Could you check a few things on this model? Use its own coordinates, in mm. Give positions to 0.01 mm unless a question says otherwise; leave off trailing zeros. Write each loop counter-clockwise with the first axis right and the second up, starting at its lowest first coordinate (ties: lowest second). Pieces come first, ordered by that corner, then holes. Notation, with made-up numbers: (-30.5, 17) - (24.5, 17) arc R20 ccw to (24.5, 36) - close; hole circle Ø10 at (-20, 88). An arc over 180 degrees is marked (long way). Write item = value, one per line.
from build123d import *
from build123d import SkipClean  # not in build123d's __all__

# Parameters (mm, degrees)
F0_R      = 3.175
F1_DEPTH  = 127
F2_DEPTH  = 76.2
F3_DEPTH  = 71.12
F4_DEPTH  = 50.8
F5_DEPTH  = 45.72
F6_DEPTH  = 25.4
F7_DEPTH  = 20.32
F9_DEPTH  = 8.89
F10_DEPTH = 3.81
F12_DEPTH = 8.89
F13_DEPTH = 3.81
F15_DEPTH = 8.89
F16_DEPTH = 3.81
F17_DEPTH = 17.78


# Not quite as in the source:
# - after a boolean that leaves OpenCascade's solid faulty, fix() repairs it


with BuildPart() as f1:
    # F0 (on Top) → F1 (new body)
    with BuildSketch(Plane.XY):
        with BuildLine():
            ThreePointArc((7.6934750952, -1.6764), (7.8287386883, -0.8430459954), (7.874, 0))
            ThreePointArc((7.874, 0), (7.8574202107, 0.5107089515), (7.8077506647, 1.0192671673))
            ThreePointArc((7.8077506647, 1.0192671673), (5.6566372636, 5.4774383491), (1.27, 7.7709057387))
            ThreePointArc((1.27, 7.7709057387), (0, 7.874), (-1.27, 7.7709057387))
            ThreePointArc((-1.27, 7.7709057387), (-7.8735779463, 0.0815249862), (-1.430634249, -7.7429426994))
            ThreePointArc((-1.430634249, -7.7429426994), (-0.0815249862, -7.8735779463), (1.27, -7.7709057387))
            ThreePointArc((1.27, -7.7709057387), (5.4195683864, -5.7121059606), (7.6934750952, -1.6764))
        make_face()
        Circle(F0_R, mode=Mode.SUBTRACT)
    extrude(amount=F1_DEPTH)

    # F0 (on Top) → F2 (join)
    with BuildSketch(Plane.XY):
        with BuildLine():
            ThreePointArc((-1.27, 7.7709057387), (0, 7.874), (1.27, 7.7709057387))
            Line((1.27, 7.7709057387), (1.27, 12.3429057387))
            Line((1.27, 12.3429057387), (-1.27, 12.3429057387))
            Line((-1.27, 12.3429057387), (-1.27, 7.7709057387))
        make_face()
    extrude(amount=F2_DEPTH)

    # F0 (on Top) → F3 (cut)
    with BuildSketch(Plane.XY):
        with BuildLine():
            ThreePointArc((-1.27, 7.7709057387), (0, 7.874), (1.27, 7.7709057387))
            Line((1.27, 7.7709057387), (1.27, 12.3429057387))
            Line((1.27, 12.3429057387), (-1.27, 12.3429057387))
            Line((-1.27, 12.3429057387), (-1.27, 7.7709057387))
        make_face()
    with SkipClean():  # cleaning this boolean's faces spoils the solid; the shape is the same uncleaned
        extrude(amount=F3_DEPTH, mode=Mode.SUBTRACT)

    # F0 (on Top) → F4 (join)
    with BuildSketch(Plane.XY):
        with BuildLine():
            ThreePointArc((7.8077506647, 1.0192671673), (7.8574202107, 0.5107089515), (7.874, 0))
            ThreePointArc((7.874, 0), (7.8287386883, -0.8430459954), (7.6934750952, -1.6764))
            Line((7.6934750952, -1.6764), (12.2654750952, -1.6764))
            Line((12.2654750952, -1.6764), (12.2654750952, 0.8636))
            Line((12.2654750952, 0.8636), (7.8077506647, 1.0192671673))
        make_face()
    extrude(amount=F4_DEPTH)

    add(f1.part.fix(), mode=Mode.REPLACE)

    # F0 (on Top) → F5 (cut)
    with BuildSketch(Plane.XY):
        with BuildLine():
            ThreePointArc((7.8077506647, 1.0192671673), (7.8574202107, 0.5107089515), (7.874, 0))
            ThreePointArc((7.874, 0), (7.8287386883, -0.8430459954), (7.6934750952, -1.6764))
            Line((7.6934750952, -1.6764), (12.2654750952, -1.6764))
            Line((12.2654750952, -1.6764), (12.2654750952, 0.8636))
            Line((12.2654750952, 0.8636), (7.8077506647, 1.0192671673))
        make_face()
    with SkipClean():  # cleaning this boolean's faces spoils the solid; the shape is the same uncleaned
        extrude(amount=F5_DEPTH, mode=Mode.SUBTRACT)

    # F0 (on Top) → F6 (join)
    with BuildSketch(Plane.XY):
        with BuildLine():
            Line((1.27, -12.3429057387), (1.27, -7.7709057387))
            ThreePointArc((1.27, -7.7709057387), (-0.0815249862, -7.8735779463), (-1.430634249, -7.7429426994))
            Line((-1.430634249, -7.7429426994), (-1.27, -12.3429057387))
            Line((-1.27, -12.3429057387), (1.27, -12.3429057387))
        make_face()
    extrude(amount=F6_DEPTH)

    add(f1.part.fix(), mode=Mode.REPLACE)

    # F0 (on Top) → F7 (cut)
    with BuildSketch(Plane.XY):
        with BuildLine():
            Line((1.27, -12.3429057387), (1.27, -7.7709057387))
            ThreePointArc((1.27, -7.7709057387), (-0.0815249862, -7.8735779463), (-1.430634249, -7.7429426994))
            Line((-1.430634249, -7.7429426994), (-1.27, -12.3429057387))
            Line((-1.27, -12.3429057387), (1.27, -12.3429057387))
        make_face()
    with SkipClean():  # cleaning this boolean's faces spoils the solid; the shape is the same uncleaned
        extrude(amount=F7_DEPTH, mode=Mode.SUBTRACT)

    # F8 (on face) → F9 (join)
    with BuildSketch(Plane.XY.offset(76.2)):
        with BuildLine():
            Line((1.27, 12.3429057387), (-1.27, 12.3429057387))
            Line((-1.27, 12.3429057387), (-1.27, 7.7709057387))
            ThreePointArc((-1.27, 7.7709057387), (0, 7.874), (1.27, 7.7709057387))
            Line((1.27, 7.7709057387), (1.27, 12.3429057387))
        make_face()
    extrude(amount=F9_DEPTH)

    # F8 (on face) → F10 (cut)
    with BuildSketch(Plane.XY.offset(76.2)):
        with BuildLine():
            Line((1.27, 12.3429057387), (-1.27, 12.3429057387))
            Line((-1.27, 12.3429057387), (-1.27, 7.7709057387))
            ThreePointArc((-1.27, 7.7709057387), (0, 7.874), (1.27, 7.7709057387))
            Line((1.27, 7.7709057387), (1.27, 12.3429057387))
        make_face()
    with SkipClean():  # cleaning this boolean's faces spoils the solid; the shape is the same uncleaned
        extrude(amount=F10_DEPTH, mode=Mode.SUBTRACT)

    # F11 (on face) → F12 (join)
    with BuildSketch(Plane.XY.offset(50.8)):
        with BuildLine():
            Line((12.2654750952, 0.8636), (7.8077506647, 1.0192671673))
            ThreePointArc((7.8077506647, 1.0192671673), (7.8669343066, -0.3334975508), (7.6934750952, -1.6764))
            Line((7.6934750952, -1.6764), (12.2654750952, -1.6764))
            Line((12.2654750952, -1.6764), (12.2654750952, 0.8636))
        make_face()
    extrude(amount=F12_DEPTH)

    # F11 (on face) → F13 (cut)
    with BuildSketch(Plane.XY.offset(50.8)):
        with BuildLine():
            Line((12.2654750952, 0.8636), (7.8077506647, 1.0192671673))
            ThreePointArc((7.8077506647, 1.0192671673), (7.8669343066, -0.3334975508), (7.6934750952, -1.6764))
            Line((7.6934750952, -1.6764), (12.2654750952, -1.6764))
            Line((12.2654750952, -1.6764), (12.2654750952, 0.8636))
        make_face()
    with SkipClean():  # cleaning this boolean's faces spoils the solid; the shape is the same uncleaned
        extrude(amount=F13_DEPTH, mode=Mode.SUBTRACT)

    # F14 (on face) → F15 (join)
    with BuildSketch(Plane.XY.offset(25.4)):
        with BuildLine():
            ThreePointArc((1.27, -7.7709057387), (-0.0815249862, -7.8735779463), (-1.430634249, -7.7429426994))
            Line((-1.430634249, -7.7429426994), (-1.27, -12.3429057387))
            Line((-1.27, -12.3429057387), (1.27, -12.3429057387))
            Line((1.27, -12.3429057387), (1.27, -7.7709057387))
        make_face()
    extrude(amount=F15_DEPTH)

    # F14 (on face) → F16 (cut)
    with BuildSketch(Plane.XY.offset(25.4)):
        with BuildLine():
            ThreePointArc((1.27, -7.7709057387), (-0.0815249862, -7.8735779463), (-1.430634249, -7.7429426994))
            Line((-1.430634249, -7.7429426994), (-1.27, -12.3429057387))
            Line((-1.27, -12.3429057387), (1.27, -12.3429057387))
            Line((1.27, -12.3429057387), (1.27, -7.7709057387))
        make_face()
    extrude(amount=F16_DEPTH, mode=Mode.SUBTRACT)

    # F0 (on Top) → F17 (cut)
    with BuildSketch(Plane.XY):
        with BuildLine():
            ThreePointArc((7.6934750952, -1.6764), (7.8287386883, -0.8430459954), (7.874, 0))
            ThreePointArc((7.874, 0), (7.8574202107, 0.5107089515), (7.8077506647, 1.0192671673))
            ThreePointArc((7.8077506647, 1.0192671673), (5.6566372636, 5.4774383491), (1.27, 7.7709057387))
            ThreePointArc((1.27, 7.7709057387), (0, 7.874), (-1.27, 7.7709057387))
            ThreePointArc((-1.27, 7.7709057387), (-7.8735779463, 0.0815249862), (-1.430634249, -7.7429426994))
            ThreePointArc((-1.430634249, -7.7429426994), (-0.0815249862, -7.8735779463), (1.27, -7.7709057387))
            ThreePointArc((1.27, -7.7709057387), (5.4195683864, -5.7121059606), (7.6934750952, -1.6764))
        make_face()
        Circle(F0_R, mode=Mode.SUBTRACT)
    extrude(amount=F17_DEPTH, mode=Mode.SUBTRACT)


solid = f1.part
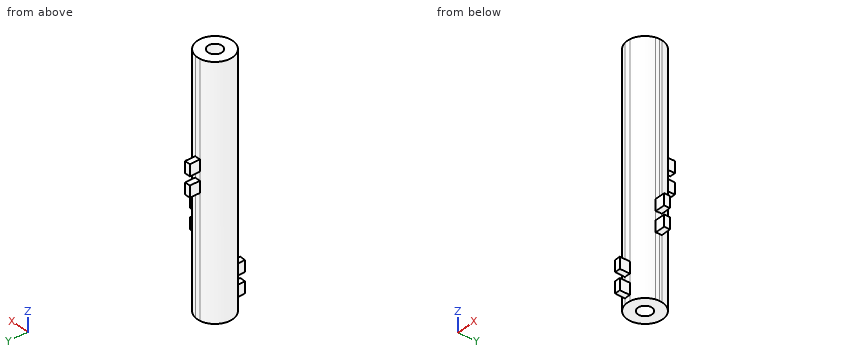
1. If we section it at D-D, the plane z = 115: Please give me the cut outline in (x, y) (3 decimals), and give its area (3 significant figures).
Filled sheet:
outline = circle Ø15.748 at (0, 0); hole circle Ø6.35 at (0, 0)
area = 163 mm2
2. I need wall thicknesses on line 1 (Y direction, x = 0, z = 42) (3 decimals); line 2 (Z direction, x = 0, y = 8.25); line 3 (Y direction, x = 1.5, z = 98). Which ranges of each line are inside material? Lowest first, please.
Filled sheet:
line_1 = -7.874 to -3.175, 3.175 to 7.874
line_2 = 71.12 to 76.2, 80.01 to 85.09
line_3 = -7.73 to -2.8, 2.8 to 7.73
3. If we section it at B-B, the plane x = 0: Please give me the cut outline in (y, z) (3 decimals).
Filled sheet:
outline = (-12.343, 20.32) - (-7.874, 20.32) - (-7.874, 17.78) - (-3.175, 17.78) - (-3.175, 127) - (-7.874, 127) - (-7.874, 34.29) - (-12.343, 34.29) - (-12.343, 29.21) - (-7.874, 29.21) - (-7.874, 25.4) - (-12.343, 25.4) - close; (3.175, 17.78) - (7.874, 17.78) - (7.874, 71.12) - (12.343, 71.12) - (12.343, 76.2) - (7.874, 76.2) - (7.874, 80.01) - (12.343, 80.01) - (12.343, 85.09) - (7.874, 85.09) - (7.874, 127) - (3.175, 127) - close
4. For pin 1 (1.5 mm diameter, centred on x = 5.5, z = 84.5, fed in from -Y); pin 2 (4 mm diameter, centred on x = 10, y = -4.5, fed in from +Z); pin 3 (2 mm diameter, centred on x = 9.5, y = -0.5, fed in from -Z); pin 4 (2.5 mm diameter, centred on y = 10, z = 83.5, fed in from -X), each with a flat end and sliding along its axis, tell me the tip position at first contact or that it passes through.
Filled sheet:
pin_1 = -6.28
pin_2 = through
pin_3 = 45.72
pin_4 = -1.27
5. If we section it at A-A, the plane y = 10.75: Please give me the cut outline in (x, z), and give its area (3 significant figures).
Filled sheet:
outline = (-1.27, 71.12) - (1.27, 71.12) - (1.27, 76.2) - (-1.27, 76.2) - close; (-1.27, 80.01) - (1.27, 80.01) - (1.27, 85.09) - (-1.27, 85.09) - close
area = 25.8 mm2
6. If we section it at C-C, the plane z = 47.5: Please give me the cut outline in (x, y) (3 decimals).
Filled sheet:
outline = (7.693, -1.676) - (12.265, -1.676) - (12.265, 0.864) - (7.808, 1.019) arc R7.874 ccw (long way) to start; hole circle Ø6.35 at (0, 0)
